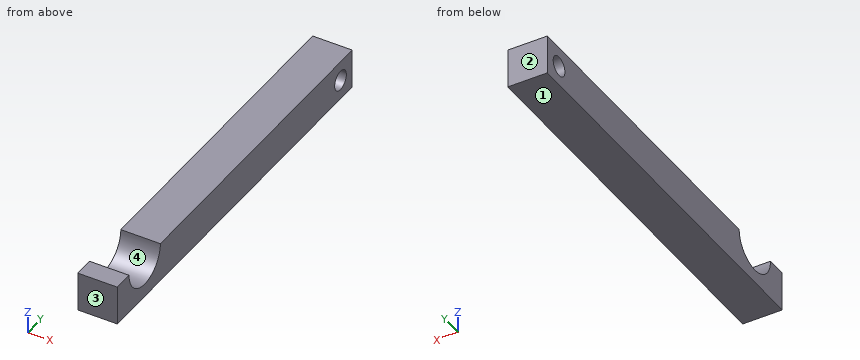
```python
from build123d import *

# Parameters (mm, degrees)
F0_W     = 38.100004
F0_H     = 38.1
F1_DEPTH = 190.5
F2_R     = 25.4
F3_DEPTH = 38.101003
F4_R     = 9.525
F5_DEPTH = 38.101003


with BuildPart() as f1:
    # F0 (on Front) → F1 (new body, symmetric)
    with BuildSketch(Plane.XZ):
        Rectangle(F0_W, F0_H)
    extrude(amount=F1_DEPTH, both=True)

    # F2 (on face) → F3 (cut, through all)
    with BuildSketch(Plane.YZ.offset(19.050002)):
        with Locations((-146.05, 19.05)):
            Circle(F2_R)
    extrude(amount=-F3_DEPTH, mode=Mode.SUBTRACT)

    # F4 (on face) → F5 (cut, through all)
    with BuildSketch(Plane.YZ.offset(19.050002)):
        with Locations((171.45, 0)):
            Circle(F4_R)
    extrude(amount=-F5_DEPTH, mode=Mode.SUBTRACT)


solid = f1.part
```
The listing builds one solid part. Answer for the finished solid, in the listing's coordinates (mm). Face numbers are marked on the shaded views. Give positions to 0.01 mm unless a question says otherwise; leave off trailing zeros. Order: outer loops, then holes, each group sorted by start corner. A loop starts at its lowest first (then second) coordinate and runs counter-clockwise, first axis right, second up.
1) Determine the mould class of the marked faces 1, 2, 3 and 4 for opening direction Y: pulls with the +Y half, pulls with the -Y half, needs draft (parallel to the pull), parting line crosses it, or undercut.
Reported:
face 1: needs draft
face 2: pulls with the +Y half
face 3: pulls with the -Y half
face 4: undercut
2) Consider line 1 along Y through (x, z) = (15, 3); line 2 along Z through (x, y) = (-16.5, 170.5); line 3 along Y through (x, z) = (-14.5, 3.5). Determine where each line is inside the solid, lowest interval first.
Reported:
line 1: y = -190.5 to -165.74, -126.36 to 162.41, 180.49 to 190.5
line 2: z = -19.05 to -9.48, 9.48 to 19.05
line 3: y = -190.5 to -166.13, -125.97 to 162.59, 180.31 to 190.5
3) Find section B-B on y = -146.05. Write down the section's boundary in (x, z), then the cut area to 3 significant figures.
Reported:
outline: (-19.05, -19.05) - (19.05, -19.05) - (19.05, -6.35) - (-19.05, -6.35) - close
area: 484 mm2
4) Find section A-A on x = -6.5. Write down the section's boundary in (y, z) (3 decimals), then the cut area to 3 significant figures.
Reported:
outline: (-190.5, -19.05) - (190.5, -19.05) - (190.5, 19.05) - (-120.65, 19.05) arc R25.4 cw to (-171.45, 19.05) - (-190.5, 19.05) - close; hole circle Ø19.05 at (171.45, 0)
area: 13,200 mm2
